The model under review builds one solid part; all positions refer to its coordinate system, in mm. Face numbers are marked on the shaded views. Round coordinates to 2 decimals unless told otherwise and drop trailing zeros. Write each loop counter-clockwise with the first axis right and the second up, starting at its lowest first coordinate (ties: lowest second). Pieces come first, ordered by that corner, then holes. Notation, with made-up numbers: (27, 36) - (40, 36) arc R21 ccw to (40, 71) - close; hole circle Ø5 at (4.25, 57.5). An arc over 180 degrees is marked (long way). Write each question's results on one line, items separated by ' | '.
```python
from build123d import *

# Parameters (mm, degrees)
SKETCH_1_R      = 1.75
EXTRUDE_1_DEPTH = 2.5
FILLET_1_R      = 0.5


with BuildPart() as part:
    # ｽｹｯﾁ1 → ﾎﾞｽ - 押し出し1 (new body)
    with BuildSketch(Plane.XY):
        Polygon((3, 0), (1.5, 2.598076211), (-1.5, 2.598076211), (-3, 0), (-1.5, -2.598076211), (1.5, -2.598076211), align=None)
        Circle(SKETCH_1_R, mode=Mode.SUBTRACT)
    extrude(amount=EXTRUDE_1_DEPTH)

    # ﾌｨﾚｯﾄ1
    fillet_1_edges = [part.edges().sort_by_distance(p)[0] for p in [
        (0, 2.598076211, 2.5),
        (-2.25, 1.299038106, 2.5),
        (-2.25, -1.299038106, 2.5),
        (0, -2.598076211, 2.5),
        (2.25, -1.299038106, 2.5),
        (2.25, 1.299038106, 2.5),
    ]]
    fillet(fillet_1_edges, radius=FILLET_1_R)


solid = part.part
```
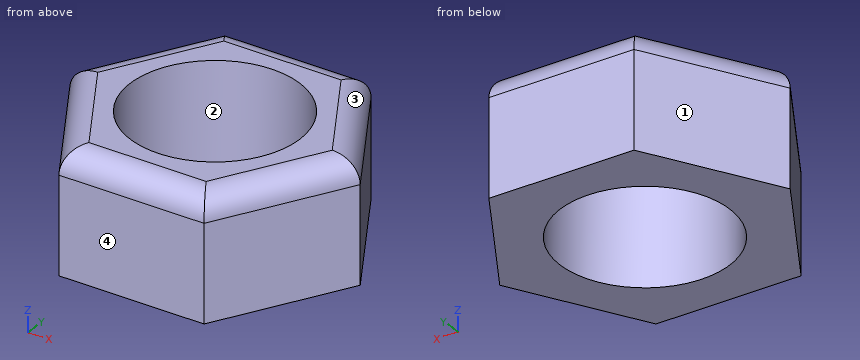
Q1. We need section B-B (z = 0.8). State the section outline as (x, y) points, plus the area to 3 significant figures.
Evaluation:
outline: (-3, 0) - (-1.5, -2.6) - (1.5, -2.6) - (3, 0) - (1.5, 2.6) - (-1.5, 2.6) - close; hole circle Ø3.5 at (0, 0) | area: 13.8 mm^2
Q2. Insertion check: P1, Ø1, axis at x = 2.5, z = 1.5, coming from the +Y side; P2, Ø3, axis at x = 2, y = -2, coming from the -Z side. Each pin has a flat end and moves straight along its axis. Give the tip position at first contact, or say it passes through.
Evaluation:
P1: stops at y = 1.73 | P2: stops at z = 0
Q3. For probe 1 along Y at (x, z) = (0, 0.95); probe 2 along Y at (x, z) = (-0.75, 2.3); probe 3 along X at (y, z) = (-1.4, 2.35), list the stretches that pass through material, from the lowest coordinate up.
Evaluation:
probe 1: y = -2.6 to -1.75, 1.75 to 2.6 | probe 2: y = -2.5 to -1.58, 1.58 to 2.5 | probe 3: x = -2.03 to -1.05, 1.05 to 2.03
Q4. We need section A-A (x = 0). State the section outline as (y, z) points, plus the area to 3 significant figures.
Evaluation:
outline: (-2.6, 0) - (-1.75, 0) - (-1.75, 2.5) - (-2.1, 2.5) arc R0.5 ccw to (-2.6, 2) - close; (1.75, 0) - (2.6, 0) - (2.6, 2) arc R0.5 ccw to (2.1, 2.5) - (1.75, 2.5) - close | area: 4.13 mm^2
Q5. The part is to be moulded in two halves that separate along X. For the marked faces 1, 2, 3 and 4, say which applies: released by +X, released by -X, zero draft, split by the parting line, or undercut.
Evaluation:
face 1: released by -X | face 2: undercut | face 3: released by +X | face 4: zero draft
Q6. We need section C-C (z = 2.25). State the section outline as (x, y) points.
Evaluation:
outline: (-2.92, 0) - (-1.46, -2.53) - (1.46, -2.53) - (2.92, 0) - (1.46, 2.53) - (-1.46, 2.53) - close; hole circle Ø3.5 at (0, 0)
